Verification items for this drawing (mm, ordinates from the low corner). Round coordinates to 2 decimals unless told otherwise and drop trailing zeros. Loops run counter-clockwise (first coordinate to the right, second up) from the corner with the lowest first, then second, coordinate; pieces in that order, holes last. Notation, with made-up numbers: (-37, -39) - (6, -39) arc R22 ccw to (6, -11) - close; hole circle Ø11 at (48.5, 75.5). An arc over 180 degrees is marked (long way). Write item = value, one per line.
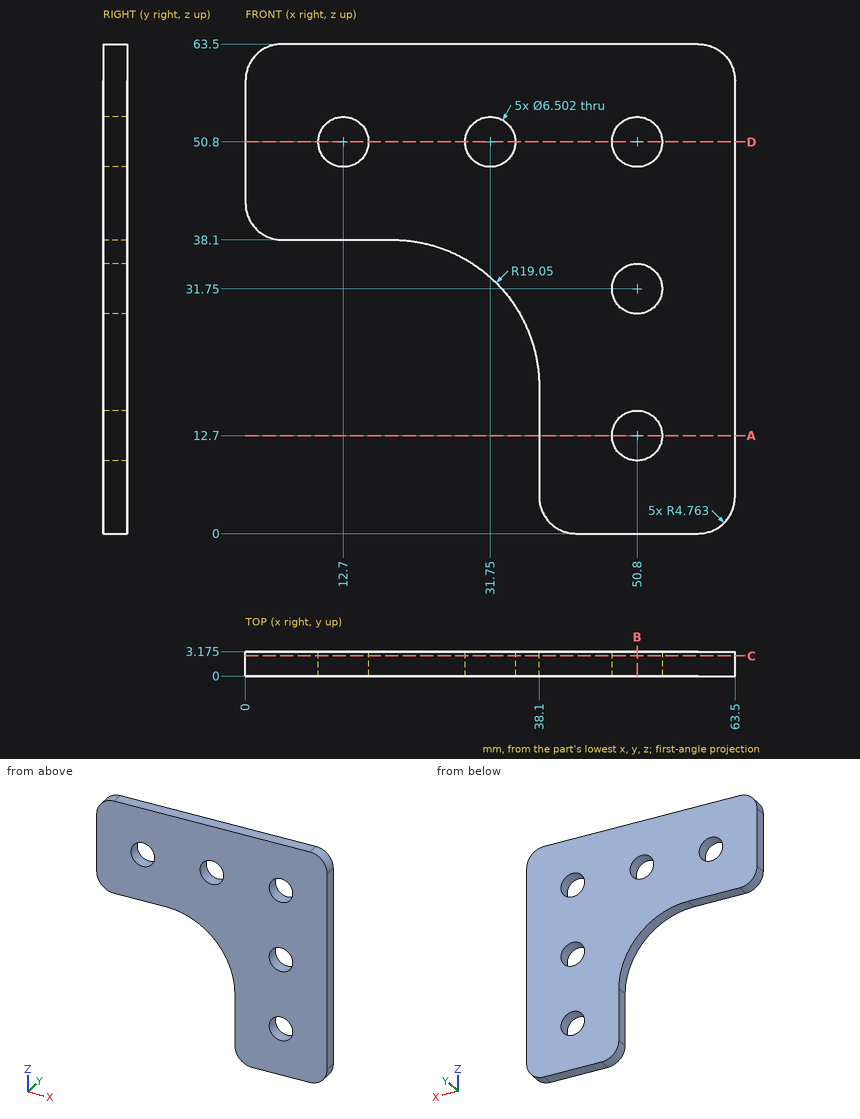
(1) Section check B-B (x = 50.8). Enter the section's corners in (y, z) (1 decimal).
Answers follow:
outline = (0, 0) - (3.2, 0) - (3.2, 9.4) - (0, 9.4) - close; (0, 16) - (3.2, 16) - (3.2, 28.5) - (0, 28.5) - close; (0, 35) - (3.2, 35) - (3.2, 47.5) - (0, 47.5) - close; (0, 54.1) - (3.2, 54.1) - (3.2, 63.5) - (0, 63.5) - close
(2) Gauge pin test, flat end, axial feed: pin 1 (1 mm diameter, centred on x = 28.5, y = 0.5, fed in from -Z) (1 decimal). Record the tip position at first contact, or that the pin passes through.
Answers follow:
pin_1 = 35.3
(3) Section check D-D (z = 50.8). Enter the section's corners in (x, y) (1 decimal).
Answers follow:
outline = (0, 0) - (9.4, 0) - (9.4, 3.2) - (0, 3.2) - close; (16, 0) - (28.5, 0) - (28.5, 3.2) - (16, 3.2) - close; (35, 0) - (47.5, 0) - (47.5, 3.2) - (35, 3.2) - close; (54.1, 0) - (63.5, 0) - (63.5, 3.2) - (54.1, 3.2) - close
(4) Section check C-C (y = 2.6). State how many separate pieces and enclosed holes the cut face has, then the cut area to 3 significant figures.
Answers follow:
separate_pieces = 1
enclosed_holes = 5
area = 2,470 mm²
(5) Scan lines: L1, parallel to Z at x = 50.8, y = 1.8; L2, parallel to Z at x = 52, y = 0.7; L3, parallel to X at y = 2.45, z = 7.5. Record each from-to range of solid material in increasing order. Write a range as [from, to].
Answers follow:
L1 = [0, 9.45], [15.95, 28.5], [35, 47.55], [54.05, 63.5]
L2 = [0, 9.68], [15.72, 28.73], [34.77, 47.78], [53.82, 63.5]
L3 = [38.1, 63.5]
(6) Section check A-A (z = 12.7). Enter the section's corners in (x, y) (1 decimal).
Answers follow:
outline = (38.1, 0) - (47.5, 0) - (47.5, 3.2) - (38.1, 3.2) - close; (54.1, 0) - (63.5, 0) - (63.5, 3.2) - (54.1, 3.2) - close
